Geometry: final body of the model. Coordinates: model frame, mm. Face numbers are marked on the shaded views. A direction names the side the tool comes from. Round coordinates to 2 decimals unless told otherwise and drop trailing zeros. Order: outer loops, then holes, each group sorted by start corner. A loop starts at its lowest first (then second) coordinate and runs counter-clockwise, first axis right, second up. Notation, with made-up numbers: M -1.75,9.5 L 11.25,9.5 A15 cw 11.25,32.5 Z; hole C 57,-20 d6. An arc over 180 degrees is marked long. Return JSON: item names as keys, results as strings. Group by question number.
Q1. Cut plane B-B on x = -12. Output: boundary loops of the cut face in (y, z), and give its area (3 significant figures).
Q2. Cut plane C-C on z = -53. Output: boundary loops of the cut face in (x, y), and give its area (3 significant figures).
Q3. Ray query, probe 1 along Y at (x, z) = (-7, -53); probe 2 along Z at (x, y) = (-4.75, 9.5); probe 3 along Z at (x, y) = (-7, 7.25). Return the intervals inside material, ascending.
Q4. Cut plane D-D on z = -37. Output: boundary loops of the cut face in (x, y), and give its area (3 significant figures).
Q5. Contact query for flat-ended pins moving along their axis: pin 1 (5 mm diameter, centred on x = -7.5, z = -47, fed in from +Y); pin 2 (1 mm diameter, centred on x = -12, z = -14.5, fed in from +Y). Output: stop coordinate, or through.
Q6. Access query for the marked faces 1, 2 and 3. Directions: +Z, -Z, +X, -X, +Y, -Y. A direction counts if a zero-diameter tool reaches every point of the face in a straight line with its end or side. Return the directions, or none.
Q7. Cut plane A-A on y = 8.5. Output: boundary loops of the cut face in (x, z).
```python
from build123d import *

# Parameters (mm, degrees)
BOSS_EXTRUDE1_DEPTH = 10


with BuildPart() as part:
    # Sketch1 → Boss-Extrude1 (new body)
    with BuildSketch(Plane.ZY.offset(4)):
        Polygon((-10, 11.5), (10, 11.5), (10, 4.5), (-10, 4.5), (-42.635866967, 4.75), (-60, 4.75), (-60, 11.25), (-14.260924963, 11.25), align=None)
        with BuildLine():
            Line((-2.049390153, 9.6), (2.049390153, 9.6))
            ThreePointArc((2.049390153, 9.6), (2.6, 8), (2.049390153, 6.4))
            Line((2.049390153, 6.4), (-2.049390153, 6.4))
            ThreePointArc((-2.049390153, 6.4), (-2.6, 8), (-2.049390153, 9.6))
        make_face(mode=Mode.SUBTRACT)
    extrude(amount=BOSS_EXTRUDE1_DEPTH)


solid = part.part
```
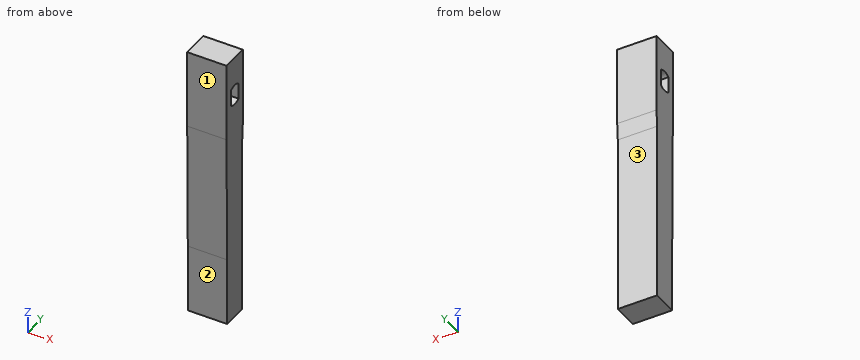
Result sheet:
{
 "1": {"outline": "M 4.5,-10 L 4.75,-42.64 L 4.75,-60 L 11.25,-60 L 11.25,-14.26 L 11.5,-10 L 11.5,10 L 4.5,10 Z; hole M 6.4,-2.05 A2.6 ccw 9.6,-2.05 L 9.6,2.05 A2.6 ccw 6.4,2.05 Z", "area": "454 mm²"},
 "2": {"outline": "M -14,4.75 L -4,4.75 L -4,11.25 L -14,11.25 Z", "area": "65.0 mm²"},
 "3": {"probe 1": "y = 4.75 to 11.25", "probe 2": "z = -60 to -2.12, 2.12 to 10", "probe 3": "z = -60 to -2.49, 2.49 to 10"},
 "4": {"outline": "M -14,4.71 L -4,4.71 L -4,11.25 L -14,11.25 Z", "area": "65.4 mm²"},
 "5": {"pin 1": "stops at y = 11.25", "pin 2": "stops at y = 11.27"},
 "6": {"face 1": "+Z, -Z, +X, -X, -Y", "face 2": "-Z, +X, -X, -Y", "face 3": "-Z, +X, -X, +Y"},
 "7": {"outline": "M -14,-60 L -4,-60 L -4,-2.55 L -14,-2.55 Z; M -14,2.55 L -4,2.55 L -4,10 L -14,10 Z"}
}
